Input: part model. Units: mm. Frame: model coordinates. Round coordinates to 2 decimals unless told otherwise and drop trailing zeros. Loops run counter-clockwise (first coordinate to the right, second up) from the corner with the lowest first, then second, coordinate; pieces in that order, holes last. Notation, with made-up numbers: (84, 41) - (103, 41) arc R7 cw to (103, 47) - close; hole circle Ø6 at (65.5, -30.5). An arc over 180 degrees is marked (long way). One line per question, with ' | ' between items. Start each with the question number.
from build123d import *

# Parameters (mm, degrees)
F0_W           = 304.8
F0_H           = 25.4
F1_DEPTH       = 101.6
F2_SIZE        = 6.35
F4_D           = 10.0838
F4_CSINK_D     = 19.8374
F4_CSINK_ANGLE = 82


with BuildPart() as f1:
    # F0 (on Front) → F1 (new body, symmetric)
    with BuildSketch(Plane.XZ):
        Rectangle(F0_W, F0_H)
    extrude(amount=F1_DEPTH, both=True)

    # F2
    f2_edges = [f1.edges().sort_by_distance(p)[0] for p in [
        (152.4, 0, -12.7),
        (-152.4, 0, -12.7),
    ]]
    chamfer(f2_edges, length=F2_SIZE)

    # F4 (through all)
    with Locations(Plane(origin=(0, 0, -12.7), x_dir=(1, 0, 0), z_dir=(0, 0, -1))):
        with Locations((-76.2, 50.8), (76.2, 50.8), (76.2, -50.8), (-76.2, -50.8)):
            CounterSinkHole(F4_D / 2, F4_CSINK_D / 2, counter_sink_angle=F4_CSINK_ANGLE)


solid = f1.part
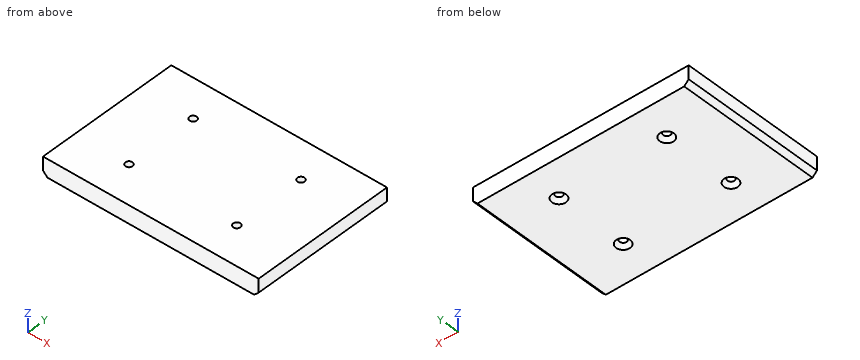
(1) Line query: line 1 along Y through (x, z) = (76.2, -0.75); line 2 along X through (y, z) = (-50.8, -0.25); line 3 along X through (y, z) = (-47, 6.75). Output: solid intervals per line, ascending. Write a range as from..to.
(2) Pin query (flat end, axial travel): P1, Ø16, axis at x = -76.2, y = 50.8, coming from the -Z side; P2, Ø9, axis at x = 76.2, y = 50.8, coming from the +Z side; P3, Ø5, axis at y = -22, z = -6.5, coming from the +X side; P4, Ø13, axis at x = -76.2, y = -50.8, coming from the -Z side. Return the tip coordinate at first contact, or that it passes through.
(3) Section A-A, the plane x = -76.2. Output: boundary loops of the cut face in (y, z), plus the area to 3 significant figures.
(4) Section B-B, the plane y = -50.8. Output: boundary loops of the cut face in (x, z).
Derived:
1) line 1: y = -101.6..-55.84, -45.76..45.76, 55.84..101.6 | line 2: x = -152.4..-81.24, -71.16..71.16, 81.24..152.4 | line 3: x = -152.4..-79.51, -72.89..72.89, 79.51..152.4
2) P1: stops at z = -10.49 | P2: passes through | P3: stops at x = 152.4 | P4: stops at z = -8.77
3) outline: (-101.6, -12.7) - (-60.72, -12.7) - (-55.84, -7.09) - (-55.84, 12.7) - (-101.6, 12.7) - close; (-45.76, -7.09) - (-40.88, -12.7) - (40.88, -12.7) - (45.76, -7.09) - (45.76, 12.7) - (-45.76, 12.7) - close; (55.84, -7.09) - (60.72, -12.7) - (101.6, -12.7) - (101.6, 12.7) - (55.84, 12.7) - close | area: 4,590 mm²
4) outline: (-152.4, -6.35) - (-146.05, -12.7) - (-86.12, -12.7) - (-81.24, -7.09) - (-81.24, 12.7) - (-152.4, 12.7) - close; (-71.16, -7.09) - (-66.28, -12.7) - (66.28, -12.7) - (71.16, -7.09) - (71.16, 12.7) - (-71.16, 12.7) - close; (81.24, -7.09) - (86.12, -12.7) - (146.05, -12.7) - (152.4, -6.35) - (152.4, 12.7) - (81.24, 12.7) - close
